Autodesk Inventor part; units mm, degrees
ref_plane "YZ Plane" through (0, 0, 0) normal (1, 0, 0) x (0, 1, 0)
ref_plane "XZ Plane" through (0, 0, 0) normal (0, 1, 0) x (-1, 0, 0)
ref_plane "XY Plane" through (0, 0, 0) normal (0, 0, 1) x (1, 0, 0)
sketch "Sketch1" plane through (0, 0, 0) normal (0, 1, 0) x (-1, 0, 0)
  line L0 (-63.5, 33.655) -> (63.5, 33.655)
  line L1 (63.5, 33.655) -> (63.5, -33.655)
  line L2 (63.5, -33.655) -> (-63.5, -33.655)
  line L3 (-63.5, -33.655) -> (-63.5, 33.655)
  line L4 (-63.5, 33.655) -> (63.5, -33.655) construction
  line L5 (63.5, 33.655) -> (-63.5, -33.655) construction
  point P0 (0, 0)
  dimension "d0" = 127
  dimension "d1" = 67.31
extrude "Extrusion1" add sketch "Sketch1" along normal mid plane 1.524
chamfer "Chamfer1" distance 19.05 angle 60 1 edges at (-63.5, 0, 33.655) measured on face at (-63.5, -0.254, 11.2183)
sketch "Sketch3" plane through (0, 0.762, 0) normal (0, 1, 0) x (1, 0, 0)
  circle A0 centre (27.7749, 27.4042) radius 1.7018
  circle A1 centre (27.7749, -23.3958) radius 1.7018
  circle A2 centre (-27.7751, -23.3958) radius 1.7018
  circle A3 centre (-27.7751, 27.4042) radius 1.7018
  point P0 (0, 0)
hole "Hole2" at (0, 0.762, 0) at (27.7749, 0.762, -27.4042) at (27.7749, 0.762, 23.3958) at (-27.7751, 0.762, 23.3958) at (-27.7751, 0.762, -27.4042) direction (0, -1, 0) diameter 3.4036 end through all
chamfer "Chamfer2" distance 19.05 angle 60 1 edges at (63.5, 0, 33.655) measured on face at (63.5, 0.254, 11.2183)
properties part number "DPLX_P022 Spark Gap Shielding Top" material "Polyethylene, High Density"
Design review of the part built by this model. Coordinates are the model's own, in mm. Give positions to 0.01 mm unless a question says otherwise; leave off trailing zeros. Order: outer loops, then holes, each group sorted by start corner. A loop starts at its lowest first (then second) coordinate and runs counter-clockwise, first axis right, second up.
1. Add section A-A, the plane x = 0. State the section outline as (y, z) points (3 decimals), then the cut area to 3 significant figures.
Solution:
outline: (-0.762, -33.655) - (0.762, -33.655) - (0.762, -1.702) - (-0.762, -1.702) - close; (-0.762, 1.702) - (0.762, 1.702) - (0.762, 33.655) - (-0.762, 33.655) - close
area: 97.4 mm2
2. For pin 1 Ø2.5 at (x, z) = (27.77, 23.4) entering from +Y, flat-tipped, find the tip position at first contact; note if it passes through.
Solution:
pin 1: passes through
3. To check wall thickness, follow L1, parallel to Z at x = 27.5, y = -0.15 (3 decimals); L2, parallel to Z at x = 0, y = -0.3 (3 decimals); L3, parallel to X at y = 0, z = 23. State the ranges of each line that lie inside material, in increasing order.
Solution:
L1: z = -33.655 to -29.084, -25.725 to 21.716, 25.075 to 33.655
L2: z = -33.655 to -1.702, 1.702 to 33.655
L3: x = -48.96 to -29.43, -26.12 to 26.12, 29.43 to 48.96
4. Mouldability with a two-part tool opening along Z and no side actions: class faces 1 (the flat face through (1, 0.762, -7)), 2 (the flat face through (46.771, -0.011, 24.263)), 3 (the cylindrical face through (0.652, -0.011, 1.572)), 4 (the cylindrical face through (26.625, -0.011, -28.658)) as +Z half, -Z half, draft (parallel to the pull), parting line (faces both ways), or undercut.
Solution:
face 1: draft
face 2: +Z half
face 3: undercut
face 4: undercut
5. Add section D-D, the plane z = 20. State the section outline as (x, y) points.
Solution:
outline: (-54.16, -0.76) - (54.16, -0.76) - (54.16, 0.76) - (-54.16, 0.76) - close
6. Add section B-B, the plane z = 0. State the section outline as (x, y) points, then the cut area to 3 significant figures.
Solution:
outline: (-63.5, -0.76) - (-1.7, -0.76) - (-1.7, 0.76) - (-63.5, 0.76) - close; (1.7, -0.76) - (63.5, -0.76) - (63.5, 0.76) - (1.7, 0.76) - close
area: 188 mm2
7. Add section C-C, the plane y = 0.15. State the section outline as (x, z) points (3 decimals).
Solution:
outline: (-63.5, -33.655) - (63.5, -33.655) - (63.5, 14.605) - (30.504, 33.655) - (-30.504, 33.655) - (-63.5, 14.605) - close; hole circle Ø3.404 at (-27.775, -27.404); hole circle Ø3.404 at (-27.775, 23.396); hole circle Ø3.404 at (0, 0); hole circle Ø3.404 at (27.775, -27.404); hole circle Ø3.404 at (27.775, 23.396)
